```python
from build123d import *

# Parameters (mm, degrees)
BOSS_EXTRUDE5_DEPTH = 15
SKETCH4_R           = 20
BOSS_EXTRUDE6_DEPTH = 2
SKETCH5_R           = 15
BOSS_EXTRUDE7_DEPTH = 41
SKETCH6_R           = 5
CUT_EXTRUDE2_DEPTH  = 100
CUT_EXTRUDE3_START  = -15
CUT_EXTRUDE3_DEPTH  = 15


with BuildPart() as part:
    # Sketch1 → Boss-Extrude5 (new body)
    with BuildSketch(Plane.XY):
        Polygon((23.094010768, 0), (11.547005384, 20), (-11.547005384, 20), (-23.094010768, 0), (-11.547005384, -20), (11.547005384, -20), align=None)
    extrude(amount=BOSS_EXTRUDE5_DEPTH)

    # Sketch4 → Boss-Extrude6 (add)
    with BuildSketch(Plane.XY.offset(15)):
        with Locations(Location((0, 0, 0), (0, 0, 150))):
            Circle(SKETCH4_R)
    extrude(amount=BOSS_EXTRUDE6_DEPTH)

    # Sketch5 → Boss-Extrude7 (add)
    with BuildSketch(Plane.XY.offset(17)):
        Circle(SKETCH5_R)
    extrude(amount=BOSS_EXTRUDE7_DEPTH)

    # Sketch6 → Cut-Extrude2 (cut)
    with BuildSketch(Plane.XY.offset(58)):
        Circle(SKETCH6_R)
    extrude(amount=-CUT_EXTRUDE2_DEPTH, mode=Mode.SUBTRACT)

    # Sketch9 → Cut-Extrude3 (cut)
    with BuildSketch(Plane.XY.offset(58).offset(CUT_EXTRUDE3_START)):
        with BuildLine():
            Line((-10, -11.180339887), (-10, 0))
            Line((-10, 0), (-10, 11.180339887))
            ThreePointArc((-10, 11.180339887), (-15, 0), (-10, -11.180339887))
        make_face()
        with BuildLine():
            Line((10, 11.180339887), (10, 0))
            Line((10, 0), (10, -11.180339887))
            ThreePointArc((10, -11.180339887), (13.693063938, -6.123724357), (15, 0))
            ThreePointArc((15, 0), (13.693063938, 6.123724357), (10, 11.180339887))
        make_face()
    extrude(amount=CUT_EXTRUDE3_DEPTH, mode=Mode.SUBTRACT)


solid = part.part
```
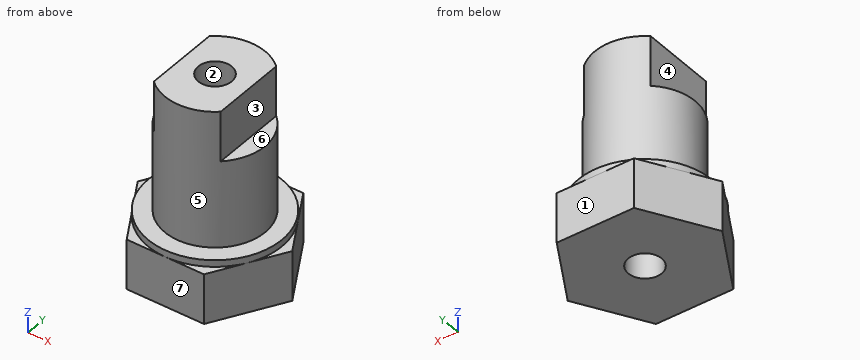
Build history of the part. All positions in model axes, mm. Face numbers are marked on the shaded views. A direction names the side the tool comes from. Round coordinates to 2 decimals unless told otherwise and drop trailing zeros. Write each loop counter-clockwise with the first axis right and the second up, starting at its lowest first coordinate (ties: lowest second). Pieces come first, ordered by that corner, then holes. Notation, with made-up numbers: (-2, 25.5) -> (21, 25.5) arc R15 ccw to (21, 30.5) -> close; hole circle Ø8 at (85.25, 53). An arc over 180 degrees is marked (long way). Put each result on its own line as item: value.
Item 1: Flat gauge pins, fed straight in: P1, Ø8, axis at x = 7, y = 16.5, coming from the +Z side; P2, Ø2, axis at x = -2, z = 38, coming from the -Y side; P3, Ø3, axis at x = 10.5, y = -17, coming from the +Z side; P4, Ø8, axis at x = 13, z = 40.5, coming from the -Y side. Where does each tip first touch, or does it go through?
Here are the results:
P1: stops at z = 58
P2: stops at y = -14.97
P3: stops at z = 17
P4: stops at y = -12
Item 2: Wall check: probe 1 along Y at (x, z) = (0, 30.5); probe 2 along Z at (x, y) = (-15.5, 8.5); probe 3 along Z at (x, y) = (14, 2). Give the ranges that are in metal, low to high. Write a range as from..to.
Here are the results:
probe 1: y = -15..-5, 5..15
probe 2: z = 0..17
probe 3: z = 0..43
Item 3: Slice it at D-D, the plane x = 13. Give the cut face in (y, z).
Here are the results:
outline: (-17.48, 0) -> (17.48, 0) -> (17.48, 15) -> (15.2, 15) -> (15.2, 17) -> (7.48, 17) -> (7.48, 43) -> (-7.48, 43) -> (-7.48, 17) -> (-15.2, 17) -> (-15.2, 15) -> (-17.48, 15) -> close
Item 4: Two-plate mould, pull along X, no slides. Class the marked faces 1, 2, 3 and 4: pulls with the +X half, pulls with the -X half, needs draft (parallel to the pull), parting line crosses it, or undercut.
Here are the results:
face 1: needs draft
face 2: undercut
face 3: pulls with the +X half
face 4: pulls with the -X half
Item 5: Tool access for the marked faces 5, 6 and 7: list every direction of +Z, -Z, +X, -X, +Y, -Y with a clear straight run to the whole face (end or side of a thin tool).
Here are the results:
face 5: +Z
face 6: +Z, +X, +Y, -Y
face 7: +Z, -Z, +X, -X, -Y
Item 6: Slice it at A-A, the plane z = 7. Give the cut face in (x, y), plus the area to 3 significant figures.
Here are the results:
outline: (-23.09, 0) -> (-11.55, -20) -> (11.55, -20) -> (23.09, 0) -> (11.55, 20) -> (-11.55, 20) -> close; hole circle Ø10 at (0, 0)
area: 1,310 mm^2
Item 7: Slice it at C-C, the plane y = -14. Give the cut face in (x, z), plus the area to 3 significant figures.
Here are the results:
outline: (-15.01, 0) -> (15.01, 0) -> (15.01, 15) -> (14.28, 15) -> (14.28, 17) -> (5.39, 17) -> (5.39, 58) -> (-5.39, 58) -> (-5.39, 17) -> (-14.28, 17) -> (-14.28, 15) -> (-15.01, 15) -> close
area: 949 mm^2
